Verification items for the finished model (mm, model axes). Round coordinates to 2 decimals unless told otherwise and drop trailing zeros. Loops run counter-clockwise (first coordinate to the right, second up) from the corner with the lowest first, then second, coordinate; pieces in that order, holes last. Notation, with made-up numbers: (-27.5, 49.5) -> (8.5, 49.5) arc R22 cw to (8.5, 84.5) -> close; hole circle Ø8 at (10.5, 72.25). An arc over 180 degrees is marked (long way). Use CSV: the item, a comma, the result in double quotes. Start each with the question number.
```python
from build123d import *

# Parameters (mm, degrees)
F2_DEPTH = 500
F3_DEPTH = 50


with BuildPart() as f2:
    # F0 (on Right) → F2 (new body, symmetric)
    with BuildSketch(Plane.YZ):
        with BuildLine():
            Line((300, -15), (300, 15))
            Line((300, 15), (-295, 15))
            ThreePointArc((-295, 15), (-298.535534, 13.535534), (-300, 10))
            Line((-300, 10), (-300, -10))
            ThreePointArc((-300, -10), (-298.535534, -13.535534), (-295, -15))
            Line((-295, -15), (300, -15))
        make_face()
    extrude(amount=F2_DEPTH, both=True)

    # F1 (on Top) → F3 (intersect, symmetric)
    with BuildSketch(Plane.XY):
        Polygon((-319.224087, 110.821992), (-189.972164, -497.260498), (462.452286, -358.5834), (333.200363, 249.49909), align=None)
    extrude(amount=F3_DEPTH, both=True, mode=Mode.INTERSECT)


solid = f2.part
```
Q1. Cross-section at B-B (x = 168). Record the boundary of the cut face in (y, z).
Q2. Cross-section at D-D (x = 254). Record the boundary of the cut face in (y, z), and give its area (3 significant figures).
Q3. Cross-section at C-C (y = 38). Record the boundary of the cut face in (x, z).
Q4. Cross-section at A-A (z = 5). Record the boundary of the cut face in (x, y).
Q5. Thickness scan on L1, parallel to Y at x = 237, z = 4.5; L2, parallel to X at y = -127, z = -3.5; L3, parallel to X at y = -21, z = 12. Record the ranges inside material, lowest first. Write a range as from..to.
Q6. Depth check by flat-ended pin: pin 1 Ø3 at (y, z) = (-206, -5.5) entering from +X; pin 2 Ø1.5 at (y, z) = (-61.5, -1) entering from -X; pin 3 Ø1 at (y, z) = (-173, 7.5) entering from -X. Enter the tip coordinate at first touch or a pass-through.
Answer list:
1,outline,"(-300, -10) arc R5 ccw to (-295, -15) -> (214.38, -15) -> (214.38, 15) -> (-295, 15) arc R5 ccw to (-300, 10) -> close"
2,outline,"(-300, -10) arc R5 ccw to (-295, -15) -> (232.66, -15) -> (232.66, 15) -> (-295, 15) arc R5 ccw to (-300, 10) -> close"
2,area,"16,000 mm2"
3,outline,"(-303.75, -15) -> (378.16, -15) -> (378.16, 15) -> (-303.75, 15) -> close"
4,outline,"(-319.22, 110.82) -> (-231.9, -300) -> (450, -300) -> (333.2, 249.5) -> close"
5,L1,"y = -300..229.05"
5,L2,"x = -268.67..413.23"
5,L3,"x = -291.2..390.7"
6,pin 1,"stops at x = 430.34"
6,pin 2,"stops at x = -282.76"
6,pin 3,"stops at x = -259"
